from build123d import *

# Parameters (mm, degrees)
F0_R     = 0.508
F1_DEPTH = 2.38125


with BuildPart() as f1:
    # F0 (on Top) → F1 (new body)
    with BuildSketch(Plane.XY):
        with BuildLine():
            ThreePointArc((0.9906, 0), (0.70046, 0.70046), (0, 0.9906))
            ThreePointArc((0, 0.9906), (-0.70046, -0.70046), (0.9906, 0))
        make_face()
        with BuildLine():
            add(Edge.make_bspline(
                [(23.077335, -0.177674), (21.532068, -0.770026), (17.205456, -2.428561), (10.097499, -5.153278), (4.534809, -7.285642), (1.753464, -8.351825)],
                knots=[3.971353, 3.971353, 3.971353, 3.971353, 8.936086, 17.872172, 26.808257, 26.808257, 26.808257, 26.808257], degree=3))
            ThreePointArc((23.077335, -0.177674), (24.566476, 2.479216), (22.225, 4.427059))
            Line((22.225, 4.427059), (0, 4.427059))
            Line((0, 4.427059), (-22.225, 4.427059))
            ThreePointArc((-22.225, 4.427059), (-24.566476, 2.479216), (-23.077335, -0.177674))
            add(Edge.make_bspline(
                [(-23.077335, -0.177674), (-21.532068, -0.770026), (-17.205456, -2.428561), (-10.097499, -5.153278), (-4.534809, -7.285642), (-1.753464, -8.351825)],
                knots=[3.971353, 3.971353, 3.971353, 3.971353, 8.936086, 17.872172, 26.808257, 26.808257, 26.808257, 26.808257], degree=3))
            ThreePointArc((-1.753464, -8.351825), (0, -8.640989), (1.753464, -8.351825))
        make_face()
        with Locations((0, -6.35)):
            Circle(F0_R, mode=Mode.SUBTRACT)
        with BuildLine():
            ThreePointArc((0.9906, 0), (-0.70046, -0.70046), (0, 0.9906))
            ThreePointArc((0, 0.9906), (0.70046, 0.70046), (0.9906, 0))
        make_face(mode=Mode.SUBTRACT)
        with Locations((-22.225, 2.045809)):
            Circle(F0_R, mode=Mode.SUBTRACT)
        with Locations((22.225, 2.045809)):
            Circle(F0_R, mode=Mode.SUBTRACT)
    extrude(amount=F1_DEPTH)


solid = f1.part
Verification items for the finished model (mm, model axes). Round coordinates to 2 decimals unless told otherwise and drop trailing zeros. Answer in a Markdown table with one row per item. Add a question column.
Q1. Release check for a two-part mould opening along X. For faces 1 (the face through (-21.756, 1.851, 1.174)), 2 (the face through (-0.02, -8.64, 1.17)), 3 (the face through (0, -2, 2.381)) record: pulls with the +X half, pulls with the -X half, needs draft (parallel to the pull), parting line crosses it, or undercut.
Q2. Material ranges on line 1 (X direction, y = 2, z = 2.1); line 2 (X direction, y = 1.75, z = 1.65); line 3 (Y direction, x = -3, z = 1.7), recorded low to high.
Q3. Section check A-A on z = 0.5. State how many separate pieces and enclosed holes the cut face has, plus the area to 3 significant figures.
Found:
| question | item | result |
|---|---|---|
| 1 | face 1 | undercut |
| 1 | face 2 | parting line crosses it |
| 1 | face 3 | needs draft |
| 2 | line 1 | x = -24.61 to -22.73, -21.72 to 21.72, 22.73 to 24.61 |
| 2 | line 2 | x = -24.59 to -22.64, -21.81 to 21.81, 22.64 to 24.59 |
| 2 | line 3 | y = -7.87 to 4.43 |
| 3 | separate pieces | 1 |
| 3 | enclosed holes | 4 |
| 3 | area | 420 mm² |
